from build123d import *

# Parameters (mm, degrees)
SKETCH1_W           = 25
SKETCH1_H           = 25
BOSS_EXTRUDE1_DEPTH = 26.6319
SKETCH2_R           = 7.96925
BOSS_EXTRUDE2_DEPTH = 21.6408
SKETCH3_R           = 3.175
BOSS_EXTRUDE3_DEPTH = 8.0899


with BuildPart() as part:
    # Sketch1 → Boss-Extrude1 (new body)
    with BuildSketch(Plane.XY):
        with Locations((12.5, 12.5)):
            Rectangle(SKETCH1_W, SKETCH1_H)
    extrude(amount=BOSS_EXTRUDE1_DEPTH)

    # Sketch2 → Boss-Extrude2 (add)
    with BuildSketch(Plane.ZY):
        with Locations((13.31595, 12.5)):
            Circle(SKETCH2_R)
    extrude(amount=BOSS_EXTRUDE2_DEPTH)

    # Sketch3 → Boss-Extrude3 (add)
    with BuildSketch(Plane(origin=(25, 0, 0), x_dir=(0, 0, -1), z_dir=(1, 0, 0))):
        with Locations((-13.31595, 12.5)):
            Circle(SKETCH3_R)
    extrude(amount=BOSS_EXTRUDE3_DEPTH)


solid = part.part
Here's how the part is built. I have some questions about the finished solid (model axes, mm). A direction names the side the tool comes from. Round coordinates to 2 decimals unless told otherwise and drop trailing zeros. Loops run counter-clockwise (first coordinate to the right, second up) from the corner with the lowest first, then second, coordinate; pieces in that order, holes last. Notation, with made-up numbers: M -34,81.5 L -8,81.5 A37 ccw -8,120.5 Z; hole C 27,-20 d5. An arc over 180 degrees is marked long. Write each question's results on one line, items separated by ' | '. Start each with the question number.
(1) I want a section at B-B (z = 8.75). Please give me the cut outline in (x, y), then the cut area to 3 significant figures.
(2) Will these pins go through, and if not, where does the flat tip stop? P1, Ø4, axis at y = 7.5, z = 8.5, coming from the +X side; P2, Ø6, axis at x = -6, z = 5.5, coming from the +Y side.
(3) On a 3-axis mill with a long thin cutter (end or side, diameter ignored), from which of +Z, -Z, +X, -X, +Y, -Y can I reach the whole of each face in a straight line? I mean faces 1 (the flat face through (25, 10, 16)), 2 (the cylindrical face through (-10.67, 14.89, 20.92)), 3 (the flat face through (-21.641, 13, 13)). Say none if no direction works.
(4) I want a section at C-C (x = -13.5). Please give me the cut outline in (y, z), then the cut area to 3 significant figures.
(5) If I drill on probe 1 along X at (y, z) = (4, 20.25); probe 2 along X at (y, z) = (13.5, 16.5); probe 3 along Y at (x, z) = (-8.5, 15.5), over which ranges is the centre line in solid material (lowest first)? Write a range as from..to.
(6) I want a section at D-D (y = 7.5). Please give me the cut outline in (x, z), then the cut area to 3 significant figures.
(7) I want a section at A-A (y = 12.5). Please give me the cut outline in (x, z), then the cut area to 3 significant figures.
Solved:
1) outline: M -21.64,5.97 L 0,5.97 L 0,0 L 25,0 L 25,25 L 0,25 L 0,19.03 L -21.64,19.03 Z | area: 908 mm²
2) P1: stops at x = 25 | P2: stops at y = 18.85
3) face 1: +X | face 2: -X | face 3: +Z, -Z, -X, +Y, -Y
4) outline: C 12.5,13.32 d15.94 | area: 200 mm²
5) probe 1: x = 0..25 | probe 2: x = -21.64..25 | probe 3: y = 4.84..20.16
6) outline: M -21.64,7.11 L 0,7.11 L 0,0 L 25,0 L 25,26.63 L 0,26.63 L 0,19.52 L -21.64,19.52 Z | area: 934 mm²
7) outline: M -21.64,5.35 L 0,5.35 L 0,0 L 25,0 L 25,10.14 L 33.09,10.14 L 33.09,16.49 L 25,16.49 L 25,26.63 L 0,26.63 L 0,21.29 L -21.64,21.29 Z | area: 1,060 mm²
